The drawing under review shows one solid part. Ordinate dimensions are in mm from its lowest x, y, z. Round coordinates to 2 decimals unless told otherwise and drop trailing zeros. Order: outer loops, then holes, each group sorted by start corner. A loop starts at its lowest first (then second) coordinate and runs counter-clockwise, first axis right, second up.
1) Consider section D-D (x = 7.25). Give the boundary of the cut face in (y, z) (1 decimal).
2) Consider section A-A (z = 108). Give the boundary of the cut face in (x, y) (1 decimal).
3) Consider section B-B (x = 117). Give the boundary of the cut face in (y, z).
4) To check wall thickness, follow L1, parallel to X at y = 7, z = 37 (1 decimal); L2, parallel to X at y = 7.25, z = 115; L3, parallel to Z at x = 170, y = 1.75 (1 decimal). State the ranges of each line that lie inside material, in increasing order.
5) Clearance check with flat-ended pins moving along their axes: P1, Ø4.5, axis at x = 100.375, z = 7.25, coming from the +Y side; P2, Ø1.5, axis at y = 4, z = 34.5, coming from the +X side (1 decimal); P3, Ø4, axis at x = 118, y = 5, coming from the +Z side; P4, Ø4, axis at y = 4.5, z = 75, coming from the +X side. State where each tip first meets the part, or that it passes through.
6) Consider section C-C (y = 8.5). Give the number of separate pieces and of enclosed holes in the cut face, then the cut area to 3 significant figures.
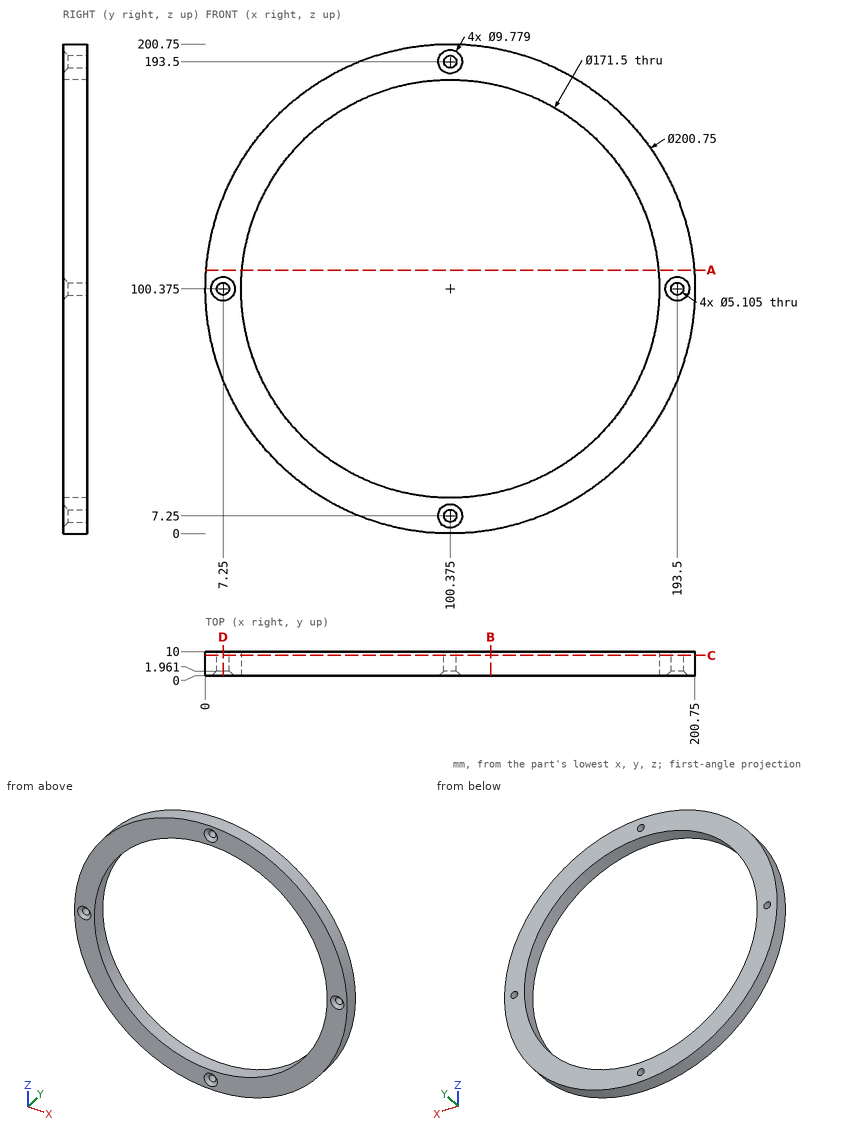
Answer below:
1. outline: (0, 62.9) - (10, 62.9) - (10, 97.8) - (2, 97.8) - (0, 95.5) - close; (0, 105.3) - (2, 102.9) - (10, 102.9) - (10, 137.8) - (0, 137.8) - close
2. outline: (0.3, 0) - (15, 0) - (15, 10) - (0.3, 10) - close; (185.8, 0) - (200.5, 0) - (200.5, 10) - (185.8, 10) - close
3. outline: (0, 1.39) - (10, 1.39) - (10, 16.25) - (0, 16.25) - close; (0, 184.5) - (10, 184.5) - (10, 199.36) - (0, 199.36) - close
4. L1: x = 22.5 to 42.6, 158.1 to 178.2
4. L2: x = 1.07 to 15.88, 184.87 to 199.68
4. L3: z = 28.1 to 50.3, 150.4 to 172.7
5. P1: passes through
5. P2: stops at x = 176.8
5. P3: stops at z = 199.53
5. P4: stops at x = 197.99
6. separate pieces: 1
6. enclosed holes: 5
6. area: 8,470 mm2
